CAD build for the part. Positions are in the model's coordinates, mm. Face numbers are marked on the shaded views. A direction names the side the tool comes from. Round coordinates to 2 decimals unless told otherwise and drop trailing zeros. Order: outer loops, then holes, each group sorted by start corner. A loop starts at its lowest first (then second) coordinate and runs counter-clockwise, first axis right, second up. Notation, with made-up numbers: M 44.5,71 L 53.5,71 A17 ccw 53.5,83 Z; hole C -13.5,54.5 d3. An arc over 180 degrees is marked long. Put each result on its own line as item: value.
```python
from build123d import *

# Parameters (mm, degrees)
SKETCH088_R             = 6
PAD064_DEPTH            = 3
SKETCH089_W             = 26
SKETCH089_H             = 3
PAD065_DEPTH            = 30
SKETCH090_R             = 2
POCKET032_DEPTH         = 30.001
SKETCH091_R             = 1
POCKET033_DEPTH         = 136.248276
POLARPATTERN013_COUNT   = 4
BODY039_PLACEMENT_ANGLE = 315


with BuildPart() as part:
    # Sketch088 → Pad064 (new body)
    with BuildSketch(Plane.XZ):
        with BuildLine():
            Line((-13, 17), (13, 17))
            Line((13, 17), (13, 0))
            ThreePointArc((-13, 0), (0, -13), (13, 0))
            Line((-13, 17), (-13, 0))
        make_face()
        Circle(SKETCH088_R, mode=Mode.SUBTRACT)
    extrude(amount=PAD064_DEPTH)

    # Sketch089 (on Face7 of Pad064) → Pad065 (join)
    with BuildSketch(Plane.XZ.offset(3)):
        with Locations((0, 15.5)):
            Rectangle(SKETCH089_W, SKETCH089_H)
    extrude(amount=PAD065_DEPTH)

    # Sketch090 (on Face5 of Pad065) → Pocket032 (cut, through all)
    with BuildSketch(Plane(origin=(0, 0, 17), x_dir=(-1, 0, 0), z_dir=(0, 0, 1))):
        with Locations((-9, 7)):
            Circle(SKETCH090_R)
        with Locations((9, 7)):
            Circle(SKETCH090_R)
        with Locations((-9, 29)):
            Circle(SKETCH090_R)
        with Locations((9, 29)):
            Circle(SKETCH090_R)
    extrude(amount=-POCKET032_DEPTH, mode=Mode.SUBTRACT)

    # Sketch091 (on Face4 of Pocket032) → Pocket033 (cut, through all)
    with BuildSketch(Plane(origin=(0, 0, 0), x_dir=(1, 0, 0), z_dir=(0, 1, 0))):
        with Locations((0, 9.5)):
            Circle(SKETCH091_R)
    pocket033 = extrude(amount=-POCKET033_DEPTH, mode=Mode.SUBTRACT)

    # PolarPattern013: Pocket033 ×4 about axis
    polarpattern013_axis = Axis((0, 0, 0), (0, 1, 0))
    for i in range(1, POLARPATTERN013_COUNT):
        add(pocket033.rotate(polarpattern013_axis, i * 360 / POLARPATTERN013_COUNT), mode=Mode.SUBTRACT)


with BuildPart() as part_1:
    # Body039 placement: moved
    add(part.part.moved(Location((53.719799, 53.720316, -7))).rotate(Axis((53.719799, 53.720316, -7), (0, 0, 1)), BODY039_PLACEMENT_ANGLE))


solid = part_1.part
```
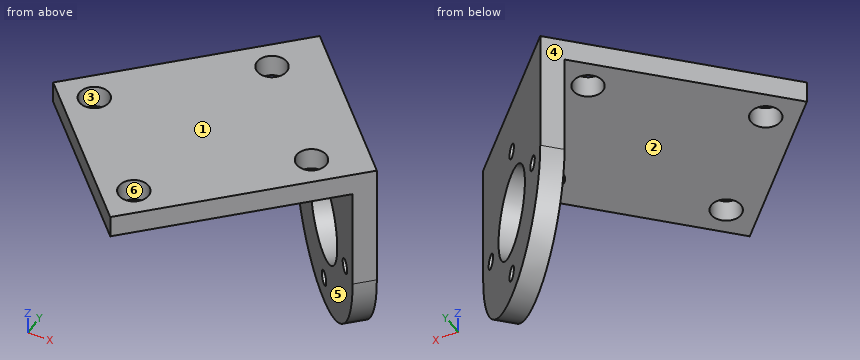
Item 1: Mould opens along Y. For the marked faces 3, 4, 5 and 6 say: pulls with the +Y half, pulls with the -Y half, needs draft (parallel to the pull), parting line crosses it, or undercut.
Answers below:
face 3: undercut
face 4: pulls with the +Y half
face 5: pulls with the -Y half
face 6: undercut
Item 2: Band-saw the part on A-A on z = -5. Give the cut face in (x, y), and give its area (3 significant figures).
Answers below:
outline: M 42.41,60.79 L 47.6,55.6 L 49.72,57.72 L 44.53,62.91 Z; M 55.6,47.6 L 60.79,42.41 L 62.91,44.53 L 57.72,49.72 Z
area: 44.1 mm²
Item 3: Probe line 1 along Z through (x, y) = (44.5, 32); line 2 along X through (y, z) = (56.5, 3.25); line 3 along X through (y, z) = (48.5, -9). List the from-to ranges inside material, lowest first. Write a range as [from, to].
Answers below:
line 1: [7, 10]
line 2: [46.7, 50.94]
line 3: [56.5, 58.94]
Item 4: Band-saw the part on C-C on x = 55. State how many separate pieces and enclosed holes the cut face has, and give its area (3 significant figures).
Answers below:
separate pieces: 3
enclosed holes: 0
area: 107 mm²
Item 5: Pin check, flat tips, straight feed: P1, Ø3.5, axis at x = 55.13, y = 42.41, coming from the +Z side; P2, Ø3, axis at x = 57.5, y = 50, coming from the -Z side; P3, Ø10, axis at y = 53, z = -16, coming from the +X side; P4, Ø10, axis at x = 38.5, y = 43.5, coming from the -Z side. Stop position of each tip, or through.
Answers below:
P1: through
P2: z = -19.43
P3: x = 59.44
P4: z = 7
Item 6: Band-saw the part on B-B on x = 39. Give the cut face in (y, z).
Answers below:
outline: M 21.77,7 L 24.94,7 L 24.94,10 L 21.77,10 Z; M 28.77,7 L 57.39,7 L 57.39,10 L 28.77,10 Z
Item 7: Tool access for the marked faces 1 and 2: list every direction of +Z, -Z, +X, -X, +Y, -Y with a clear straight run to the whole face (end or side of a thin tool).
Answers below:
face 1: +Z, +X, -X, +Y, -Y
face 2: -Z, -X, -Y
Item 8: Band-saw the part on D-D on z = 0.25. Give the cut face in (x, y), and give its area (3 significant figures).
Answers below:
outline: M 42.41,60.79 L 60.79,42.41 L 62.91,44.53 L 44.53,62.91 Z
area: 78.0 mm²
